Design review of the part shown in the three views and the two pictorial views. Dimensions are in mm from the part's minimum x, y and z. A direction names the side the tool comes from. Round coordinates to 2 decimals unless told otherwise and drop trailing zeros. Order: outer loops, then holes, each group sorted by start corner. A loop starts at its lowest first (then second) coordinate and runs counter-clockwise, first axis right, second up. Notation, with made-up numbers: (-14, 42.25) - (-1, 42.25) arc R11 cw to (-1, 63.25) - close; hole circle Ø11 at (-38.5, -37). An arc over 180 degrees is marked (long way). Use CSV: the item, a comma, the result in double quotes.
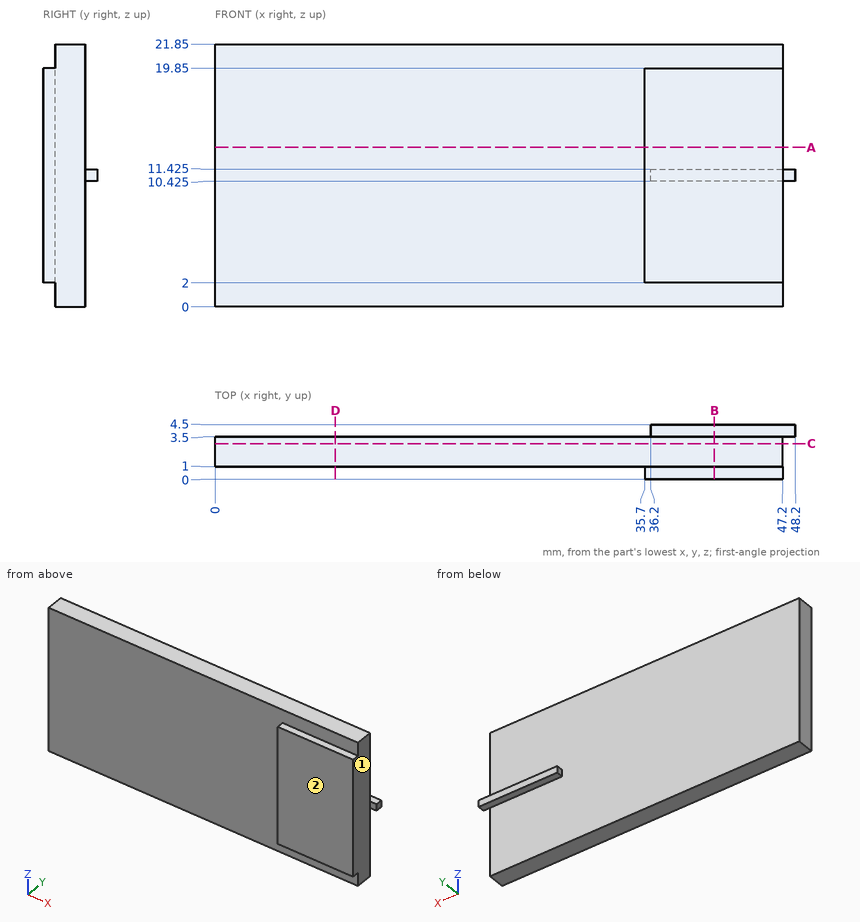
1) We need section A-A (z = 13.25). Give the boundary of the cut face in (x, y).
Data:
outline,"(0, 1) - (35.7, 1) - (35.7, 0) - (47.2, 0) - (47.2, 3.5) - (0, 3.5) - close"
2) For the marked faces 1 and 2, list the 3-axis set-ups (+Z, -Z, +X, -X, +Y, -Y) from which the entire face can be reached by the end or side of a thin tool; tool diameter is ignored.
Data:
face 1,"+Z, -Z, +X, -Y"
face 2,"+Z, -Z, +X, -X, -Y"
3) We need section C-C (y = 2.95). Give the boundary of the cut face in (x, z).
Data:
outline,"(0, 0) - (47.2, 0) - (47.2, 21.85) - (0, 21.85) - close"
4) We need section D-D (x = 10). Give the boundary of the cut face in (y, z), then the cut area to 3 significant figures.
Data:
outline,"(1, 0) - (3.5, 0) - (3.5, 21.85) - (1, 21.85) - close"
area,"54.6 mm2"
5) We need section B-B (x = 41.5). Give the boundary of the cut face in (y, z) (3 decimals), then the cut area to 3 significant figures.
Data:
outline,"(0, 2) - (1, 2) - (1, 0) - (3.5, 0) - (3.5, 10.425) - (4.5, 10.425) - (4.5, 11.425) - (3.5, 11.425) - (3.5, 21.85) - (1, 21.85) - (1, 19.85) - (0, 19.85) - close"
area,"73.5 mm2"
6) To check wall thickness, follow L1, parallel to X at y = 1.85, z = 2.25; L2, parallel to Z at x = 37, y = 0.95; L3, parallel to Y at x = 25, z = 9.75. State the ranges of each line that lie inside material, in increasing order. Write a range as from..to.
Data:
L1,"x = 0..47.2"
L2,"z = 2..19.85"
L3,"y = 1..3.5"
7) Insertion check: pin 1 Ø1.5 at (x, z) = (17.5, 13) entering from +Y; pin 2 Ø1 at (y, z) = (1, 14.5) entering from +X; pin 3 Ø6.5 at (x, z) = (21.5, 8.5) entering from -Y. Each pin has a flat end and moves straight along its axis. Give the tip position at first contact, or say it passes through.
Data:
pin 1,"stops at y = 3.5"
pin 2,"stops at x = 47.2"
pin 3,"stops at y = 1"
